Part print with two shaded views. Sizes in mm from the minimum x, y, z corner. Round coordinates to 2 decimals unless told otherwise and drop trailing zeros. Order: outer loops, then holes, each group sorted by start corner. A loop starts at its lowest first (then second) coordinate and runs counter-clockwise, first axis right, second up. Notation, with made-up numbers: M -39,-14 L 19,-14 A21 ccw 19,22 Z; hole C -14,65 d2. An arc over 180 degrees is marked long. One line per question, with ' | ' between items.
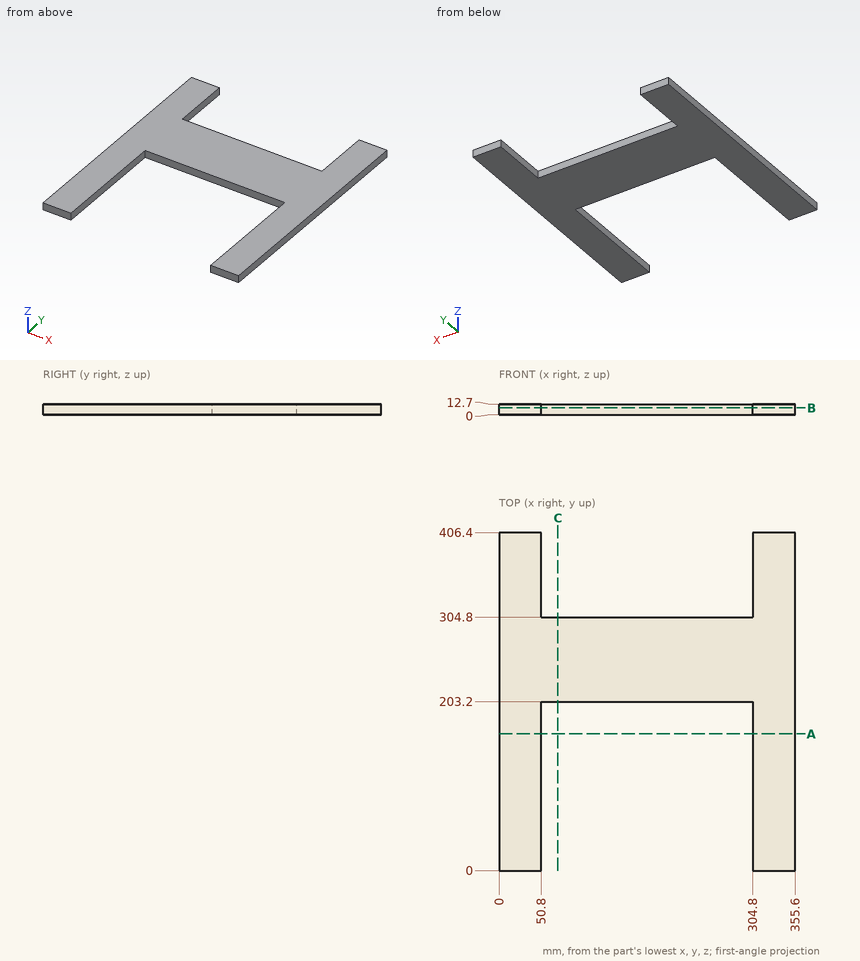
1) Saw through at C-C (x = 70.5). List the corners of the cut face in (y, z), plus the area to 3 significant figures.
The answers:
outline: M 203.2,0 L 304.8,0 L 304.8,12.7 L 203.2,12.7 Z | area: 1,290 mm²
2) Saw through at B-B (z = 8). List the corners of the cut face in (x, y), plus the area to 3 significant figures.
The answers:
outline: M 0,0 L 50.8,0 L 50.8,203.2 L 304.8,203.2 L 304.8,0 L 355.6,0 L 355.6,406.4 L 304.8,406.4 L 304.8,304.8 L 50.8,304.8 L 50.8,406.4 L 0,406.4 Z | area: 67,100 mm²
3) Probe line 1 (X direction, y = 146.5, z = 12); line 2 (Y direction, x = 230, z = 5.5). List the from-to ranges inside material, lowest first. Write a range as [from, to].
The answers:
line 1: x = [0, 50.8], [304.8, 355.6] | line 2: y = [203.2, 304.8]
4) Drop a flat-ended pin along its axis: pin 1 (2 mm diameter, centred on x = 302, z = 7.5, fed in from +Y). Give the stop position or say it passes through.
The answers:
pin 1: stops at y = 304.8
5) Saw through at A-A (y = 164.5). List the corners of the cut face in (x, z).
The answers:
outline: M 0,0 L 50.8,0 L 50.8,12.7 L 0,12.7 Z; M 304.8,0 L 355.6,0 L 355.6,12.7 L 304.8,12.7 Z
